Check sheet for the modelled part. Datum: model origin and axes. Units: mm. A direction names the side the tool comes from. Give positions to 0.01 mm unless a question says otherwise; leave off trailing zeros. Write each loop counter-clockwise with the first axis right and the second up, starting at its lowest first coordinate (ties: lowest second). Pieces come first, ordered by that corner, then holes. Notation, with made-up numbers: (81.5, -34.5) -> (131.5, -34.5) arc R26 ccw to (131.5, -9.5) -> close; hole circle Ø2 at (21.5, -16). An arc over 180 degrees is marked (long way). Answer as a JSON object with one key per item and string values.
from build123d import *

# Parameters (mm, degrees)
F0_W      = 6.35
F0_H      = 6.35
F1_DEPTH  = 101.6
F2_W      = 6.35
F2_H      = 6.35
F3_DEPTH  = 101.6
F4_W      = 6.35
F4_H      = 6.35
F5_DEPTH  = 95.25
F6_W      = 6.35
F6_H      = 6.35
F7_DEPTH  = 99.822
F8_W      = 6.35
F8_H      = 6.35
F9_DEPTH  = 101.6
F10_W     = 6.35
F10_H     = 6.35
F11_DEPTH = 101.6
F12_W     = 6.35
F12_H     = 6.35
F13_DEPTH = 97.536
F14_W     = 6.35
F14_H     = 6.35
F15_DEPTH = 95.25
F16_W     = 6.35
F16_H     = 6.35
F17_DEPTH = 96.52
F18_W     = 6.35
F18_H     = 6.35
F19_DEPTH = 101.6
F20_W     = 6.35
F20_H     = 6.35
F21_DEPTH = 92.202
F22_W     = 6.35
F22_H     = 6.35
F23_DEPTH = 97.282
F25_R     = 2.462176
F28_DEPTH = 89.916
F26_R     = 2.454167
F29_DEPTH = 91.186
F30_R     = 2.719492
F31_DEPTH = 91.186
F27_R     = 1.799115
F32_DEPTH = 92.456
F36_R     = 2.278566
F35_W     = 4.342094
F35_H     = 3.394946
F33_R     = 2.005298
F34_R     = 1.740829
F37_DEPTH = 95.25
F24_R     = 2.104729
F38_R     = 1.742329
F39_R     = 1.924697
F39_R_2   = 1.834859
F40_DEPTH = 95.25
F41_R     = 2.666191
F42_R     = 1.946965
F43_R     = 2.600414
F43_R_2   = 1.988129
F44_DEPTH = 95.25


with BuildPart() as f1:
    # F0 (on Top) → F1 (new body)
    with BuildSketch(Plane.XY):
        with Locations((-49.143255, 53.25494)):
            Rectangle(F0_W, F0_H)
    extrude(amount=F1_DEPTH)

    # F2 (on face) → F3 (join)
    with BuildSketch(Plane.XZ.offset(-50.07994)):
        with Locations((-49.143255, 3.175)):
            Rectangle(F2_W, F2_H)
    extrude(amount=F3_DEPTH)

    # F4 (on face) → F5 (join)
    with BuildSketch(Plane.XY.offset(6.35)):
        with Locations((-49.143255, -48.34506)):
            Rectangle(F4_W, F4_H)
    extrude(amount=F5_DEPTH)

    # F6 (on face) → F7 (join)
    with BuildSketch(Plane.XZ.offset(-50.07994)):
        with Locations((-49.143255, 98.425)):
            Rectangle(F6_W, F6_H)
    extrude(amount=F7_DEPTH)

    # F8 (on face) → F9 (join)
    with BuildSketch(Plane.YZ.offset(-45.968255)):
        with Locations((53.25494, 3.175)):
            Rectangle(F8_W, F8_H)
    extrude(amount=F9_DEPTH)

    # F10 (on face) → F11 (join)
    with BuildSketch(Plane.YZ.offset(-45.968255)):
        with Locations((-48.34506, 3.175)):
            Rectangle(F10_W, F10_H)
    extrude(amount=F11_DEPTH)

    # F12 (on face) → F13 (join)
    with BuildSketch(Plane.XZ.offset(-50.07994)):
        with Locations((52.456745, 3.175)):
            Rectangle(F12_W, F12_H)
    extrude(amount=F13_DEPTH)

    # F14 (on face) → F15 (join)
    with BuildSketch(Plane.XY.offset(6.35)):
        with Locations((52.456745, -48.34506)):
            Rectangle(F14_W, F14_H)
    extrude(amount=F15_DEPTH)

    # F16 (on face) → F17 (join)
    with BuildSketch(Plane(origin=(49.281745, 0, 0), x_dir=(0, -1, 0), z_dir=(-1, 0, 0))):
        with Locations((48.34506, 98.425)):
            Rectangle(F16_W, F16_H)
    extrude(amount=F17_DEPTH)

    # F18 (on face) → F19 (join)
    with BuildSketch(Plane.YZ.offset(-45.968255)):
        with Locations((53.25494, 98.425)):
            Rectangle(F18_W, F18_H)
    extrude(amount=F19_DEPTH)

    # F20 (on face) → F21 (join)
    with BuildSketch(Plane(origin=(0, 0, 95.25), x_dir=(1, 0, 0), z_dir=(0, 0, -1))):
        with Locations((52.456745, -53.25494)):
            Rectangle(F20_W, F20_H)
    extrude(amount=F21_DEPTH)

    # F22 (on face) → F23 (join)
    with BuildSketch(Plane(origin=(0, -45.17006, 0), x_dir=(-1, 0, 0), z_dir=(0, 1, 0))):
        with Locations((-52.456745, 98.425)):
            Rectangle(F22_W, F22_H)
    extrude(amount=F23_DEPTH)

    # F25 (on face) → F28 (join)
    with BuildSketch(Plane.XY.offset(6.35)):
        with Locations((52.8422, 39.234169)):
            Circle(F25_R)
    extrude(amount=F28_DEPTH)

    # F26 (on face) → F29 (join)
    with BuildSketch(Plane.XY.offset(6.35)):
        with Locations((52.487113, 6.482171)):
            Circle(F26_R)
    extrude(amount=F29_DEPTH)

    # F30 (on face) → F31 (join)
    with BuildSketch(Plane.XY.offset(6.35)):
        with Locations((52.195251, -34.391616)):
            Circle(F30_R)
    extrude(amount=F31_DEPTH)

    # F27 (on face) → F32 (join)
    with BuildSketch(Plane.XY.offset(6.35)):
        with Locations((52.82953, -17.009571)):
            Circle(F27_R)
    extrude(amount=F32_DEPTH)

    # F36 (on face) + F35 (on face) + F33 (on face) + F34 (on face) → F37 (join)
    with BuildSketch(Plane.XY.offset(6.35)):
        with Locations((-37.470926, -47.676794)):
            Circle(F36_R)
    with BuildSketch(Plane.XY.offset(6.35)):
        with Locations((-19.814698, -49.322378)):
            Rectangle(F35_W, F35_H)
    with BuildSketch(Plane.XY.offset(6.35)):
        with Locations((31.782679, -48.681542)):
            Circle(F33_R)
    with BuildSketch(Plane.XY.offset(6.35)):
        with Locations((7.43586, -48.585169)):
            Circle(F34_R)
    extrude(amount=F37_DEPTH)

    # F24 (on face) + F38 (on face) + F39 (on face) → F40 (join)
    with BuildSketch(Plane.XY.offset(6.35)):
        with Locations((-48.291616, 33.099722)):
            Circle(F24_R)
    with BuildSketch(Plane.XY.offset(6.35)):
        with Locations((-48.953682, 16.539522)):
            Circle(F38_R)
    with BuildSketch(Plane.XY.offset(6.35)):
        with Locations((-48.339192, -1.503361)):
            Circle(F39_R)
        with Locations((-48.496198, -20.61478)):
            Circle(F39_R_2)
    extrude(amount=F40_DEPTH)

    # F41 (on face) + F42 (on face) + F43 (on face) → F44 (join)
    with BuildSketch(Plane.XY.offset(6.35)):
        with Locations((34.443427, 53.185832)):
            Circle(F41_R)
    with BuildSketch(Plane.XY.offset(6.35)):
        with Locations((15.748598, 52.282806)):
            Circle(F42_R)
    with BuildSketch(Plane.XY.offset(6.35)):
        with Locations((-27.372204, 53.411223)):
            Circle(F43_R)
        with Locations((-4.064131, 52.890539)):
            Circle(F43_R_2)
    extrude(amount=F44_DEPTH)


solid = f1.part
1. Sectioned sample at C-C, the plane z = 11. State how many separate pieces and enclosed holes the cut face has, plus the area to 3 significant figures.
Determined:
{"separate pieces": "20", "enclosed holes": "0", "area": "399 mm^2"}
2. Go/stop test with flat-tipped pins: P1, Ø6, axis at x = 34, z = 44.5, coming from the +Y side; P2, Ø7, axis at x = -12.5, y = -49, coming from the -Z side; P3, Ø8, axis at y = 40.5, z = 15.5, coming from the -X side; P4, Ø4, axis at y = 9, z = 24.5, coming from the -X side. Record where each tip stops, or that it passes through.
Determined:
{"P1": "y = 55.85", "P2": "z = 0", "P3": "x = 50.38", "P4": "x = 50.09"}
3. Access from +Z, -Z, +X, -X, +Y, -Y to the whole of each face (thin tool, end or side, straight path). Record for faces 1 (the face through (53, -45.17, 50)), 2 (the face through (-45.968, 3, 3)), 3 (the face through (32.86, -46.99, 50.18)).
Determined:
{"face 1": "+X, -X", "face 2": "+Z, -Z", "face 3": "none"}
4. Sectioned sample at A-A, the plane x = 2. Enter the section's corners in (y, z).
Determined:
{"outline": "(-51.52, 0) -> (-45.17, 0) -> (-45.17, 6.35) -> (-51.52, 6.35) -> close; (-51.52, 95.25) -> (-45.17, 95.25) -> (-45.17, 101.6) -> (-51.52, 101.6) -> close; (50.08, 0) -> (56.43, 0) -> (56.43, 6.35) -> (50.08, 6.35) -> close; (50.08, 95.25) -> (56.43, 95.25) -> (56.43, 101.6) -> (50.08, 101.6) -> close"}
5. Mould release check, pull along Z, two halves, no side actions. Record for faces 4 (the face through (-47, 3, 0)), 5 (the face through (1, -45.17, 3)), 6 (the face through (1, 53, 95.25)): released by +Z, released by -Z, zero draft, split by the parting line, or undercut.
Determined:
{"face 4": "released by -Z", "face 5": "zero draft", "face 6": "undercut"}
6. Scan lines: L1, parallel to X at y = -22.5, z = 4.5; L2, parallel to Y at x = 17.5, z = 96.5; L3, parallel to X at y = 32, z = 78.5. Record each from-to range of solid material in increasing order. Write a range as [from, to].
Determined:
{"L1": "[-52.32, -45.97], [49.28, 55.63]", "L2": "[-51.52, -45.17], [50.08, 56.43]", "L3": "[-50.09, -46.5]"}
7. Sectioned sample at B-B, the plane y = 24. Enter the section's corners in (x, z).
Determined:
{"outline": "(-52.32, 0) -> (-45.97, 0) -> (-45.97, 6.35) -> (-52.32, 6.35) -> close; (-52.32, 95.25) -> (-45.97, 95.25) -> (-45.97, 101.6) -> (-52.32, 101.6) -> close; (49.28, 0) -> (55.63, 0) -> (55.63, 6.35) -> (49.28, 6.35) -> close; (49.28, 95.25) -> (55.63, 95.25) -> (55.63, 101.6) -> (49.28, 101.6) -> close"}
